```python
from build123d import *

# Parameters (mm, degrees)
SKETCH1_R           = 6
SKETCH1_R_2         = 5
BOSS_EXTRUDE1_DEPTH = 3
SKETCH2_R           = 6
BOSS_EXTRUDE2_DEPTH = 2
FILLET1_R           = 2


with BuildPart() as part:
    # Sketch1 → Boss-Extrude1 (new body)
    with BuildSketch(Plane(origin=(0, 0, 0), x_dir=(1, 0, 0), z_dir=(0, 1, 0))):
        with Locations((-0.477560777, 0)):
            Circle(SKETCH1_R)
        with Locations((-0.477560777, 0)):
            Circle(SKETCH1_R_2, mode=Mode.SUBTRACT)
    extrude(amount=BOSS_EXTRUDE1_DEPTH)

    # Sketch2 → Boss-Extrude2 (add)
    with BuildSketch(Plane(origin=(0, 3, 0), x_dir=(1, 0, 0), z_dir=(0, 1, 0))):
        with Locations((-0.477560777, 0)):
            Circle(SKETCH2_R)
    extrude(amount=BOSS_EXTRUDE2_DEPTH)

    # Fillet1
    fillet1_edges = [part.edges().sort_by_distance(p)[0] for p in [
        (-6.477560777, 5, 0),
    ]]
    fillet(fillet1_edges, radius=FILLET1_R)


solid = part.part
```
For this review, take the finished solid that the model builds, in its own axes (mm). Round coordinates to 2 decimals unless told otherwise and drop trailing zeros. Loops run counter-clockwise (first coordinate to the right, second up) from the corner with the lowest first, then second, coordinate; pieces in that order, holes last.
(1) Wall thickness on line 1 along X through (y, z) = (2.25, 0); line 2 along X through (y, z) = (2.35, 3.5); line 3 along Y through (x, z) = (2.5, 0.75): over which ranges is each line inside the solid? List them lowest first.
Returned:
line 1: x = -6.48 to -5.48, 4.52 to 5.52
line 2: x = -5.35 to -4.05, 3.09 to 4.4
line 3: y = 3 to 5
(2) We need section D-D (y = 3.3). Give the boundary of the cut face in (x, z).
Returned:
outline: circle Ø11.95 at (-0.48, 0)
(3) We need section C-C (y = 4.25). Give the boundary of the cut face in (x, z), plus the area to 3 significant figures.
Returned:
outline: circle Ø11.12 at (-0.48, 0)
area: 97.2 mm2
(4) We need section A-A (z = 0). Give the boundary of the cut face in (x, y).
Returned:
outline: (-6.48, 0) - (-5.48, 0) - (-5.48, 3) - (4.52, 3) - (4.52, 0) - (5.52, 0) - (5.52, 3) arc R2 ccw to (3.52, 5) - (-4.48, 5) arc R2 ccw to (-6.48, 3) - close
(5) We need section B-B (y = 1.8). Give the boundary of the cut face in (x, z).
Returned:
outline: circle Ø12 at (-0.48, 0); hole circle Ø10 at (-0.48, 0)
(6) Clearance check with flat-ended pins moving along their axes: P1, Ø2, axis at y = 2.5, z = 4.5, coming from the +X side; P2, Ø1, axis at x = -2.5, y = 0.5, coming from the +Z side; P3, Ø2, axis at y = 3.5, z = 3, coming from the -X side. State where each tip first meets the part, or that it passes through.
Returned:
P1: stops at x = 4.4
P2: stops at z = 5.8
P3: stops at x = -6.11
(7) Mouldability with a two-part tool opening along Z and no side actions: class faces 1 (the cylindrical face through (-5.2, 1.5, 3.7)), 2 (the flat face through (-2, 0, -5)), 3 (the cylindrical face through (-4.445, 1.479, 3.042)), 4 (the flat face through (-1, 3, 0)) as released by +Z, released by -Z, zero draft, split by the parting line, or undercut.
Returned:
face 1: split by the parting line
face 2: zero draft
face 3: undercut
face 4: undercut
